Geometry check sheet. Reference: the model listing, model coordinates, mm. Face numbers are marked on the shaded views. A direction names the side the tool comes from. Round coordinates to 2 decimals unless told otherwise and drop trailing zeros. Order: outer loops, then holes, each group sorted by start corner. A loop starts at its lowest first (then second) coordinate and runs counter-clockwise, first axis right, second up. Notation, with made-up numbers: (8, 55) -> (30, 55) arc R26 cw to (30, 93) -> close; hole circle Ø5 at (61, 41). An arc over 180 degrees is marked (long way). Use a Markdown table: item, result. Add a question column.
Item 1: Material ranges on probe 1 along Y at (x, z) = (-0.25, 0); probe 2 along Y at (x, z) = (-1.5, -1.5); probe 3 along Z at (x, y) = (0, 14.25), recorded low to high. Write a range as [from, to].
Item 2: Sectioned sample at A-A, the plane y = 19.75. Record the cut outline in (x, z).
Item 3: Sectioned sample at B-B, the plane x = 0.75. Record the cut outline in (y, z).
Item 4: Set-up check for the marked faces 1 and 2: record each of +Z, -Z, +X, -X, +Y, -Y from which the full face is reachable in a straight line by a thin tool's end or side.
Item 5: Sectioned sample at C-C, the plane y = 11.5. Record the cut outline in (x, z), and give its area (3 significant figures).
Item 6: Gauge pin test, flat ends, axial feed: pin 1 Ø4 at (y, z) = (3.5, 2) entering from +X; pin 2 Ø1 at (x, y) = (0, 8) entering from +Z; pin 3 Ø1.8 at (x, z) = (-0.5, 0.5) entering from +Y. Record the tip position at first contact, or that the pin passes through.
Item 7: Sectioned sample at D-D, the plane z = 1.5. Record the cut outline in (x, y), and give its area (3 significant figures).
Item 8: Mould release check, pull along X, two halves, no side actions. Record for the marked faces 3, 4 and 5: pulls with the +X half, pulls with the -X half, needs draft (parallel to the pull), parting line crosses it, or undercut.
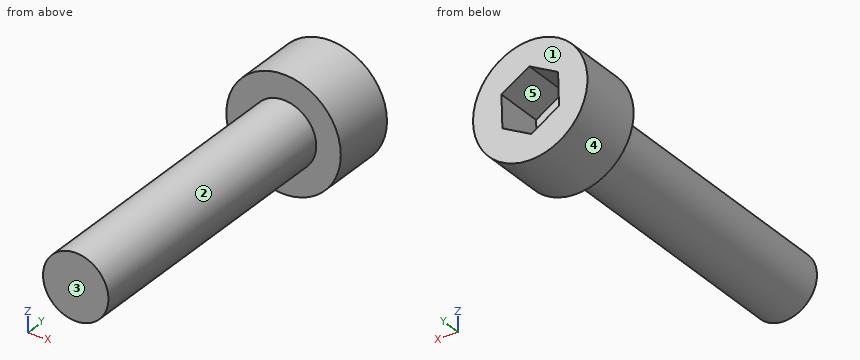
Autodesk Inventor part; units mm, degrees
ref_plane "YZ Plane" through (0, 0, 0) normal (1, 0, 0) x (0, 1, 0)
ref_plane "XZ Plane" through (0, 0, 0) normal (0, 1, 0) x (-1, 0, 0)
ref_plane "XY Plane" through (0, 0, 0) normal (0, 0, 1) x (1, 0, 0)
sketch "Sketch1" plane through (0, 0, 0) normal (0, 1, 0) x (-1, 0, 0)
  circle A0 centre (0, 0) radius 2
  dimension "d0" = 4
extrude "Extrusion1" add sketch "Sketch1" along normal blind 18
sketch "Sketch2" plane through (0, 18, 0) normal (0, 1, 0) x (1, 0, 0)
  circle A0 centre (0, 0) radius 3.5
  dimension "d5" = 7
thread "Thread1"
extrude "Extrusion2" add sketch "Sketch2" along normal blind 4
sketch "Sketch3" plane through (0, 22, 0) normal (0, 1, 0) x (1, 0, 0)
  circle A0 centre (0, 0) radius 3.5
  circle A1 centre (0, 0) radius 2
  line L0 (-1.7603, 0.9494) -> (-0.058, 1.9992)
  line L1 (-0.058, 1.9992) -> (1.7023, 1.0498)
  line L2 (1.7023, 1.0498) -> (1.7603, -0.9494)
  line L3 (1.7603, -0.9494) -> (0.058, -1.9992)
  line L4 (0.058, -1.9992) -> (-1.7023, -1.0498)
  line L5 (-1.7023, -1.0498) -> (-1.7603, 0.9494)
extrude "Extrusion3" cut sketch "Sketch3" against normal blind 3 contours L2 L3 L4 L5 L0 L1
properties part number "M4_18mm" material "Steel, Alloy"
Found:
| question | item | result |
|---|---|---|
| 1 | probe 1 | y = [0, 19] |
| 1 | probe 2 | y = [18, 22] |
| 1 | probe 3 | z = [-2, 2] |
| 2 | outline | circle Ø7 at (0, 0); hole (-1.76, -0.95) -> (-0.06, -2) -> (1.7, -1.05) -> (1.76, 0.95) -> (0.06, 2) -> (-1.7, 1.05) -> close |
| 3 | outline | (0, -1.85) -> (18, -1.85) -> (18, -3.42) -> (22, -3.42) -> (22, -1.56) -> (19, -1.56) -> (19, 1.57) -> (22, 1.57) -> (22, 3.42) -> (18, 3.42) -> (18, 1.85) -> (0, 1.85) -> close |
| 4 | face 1 | +Z, -Z, +X, -X, +Y |
| 4 | face 2 | -Y |
| 5 | outline | circle Ø4 at (0, 0) |
| 5 | area | 12.6 mm2 |
| 6 | pin 1 | stops at x = 2 |
| 6 | pin 2 | stops at z = 2 |
| 6 | pin 3 | stops at y = 19 |
| 7 | outline | (-3.16, 18) -> (-1.32, 18) -> (-1.32, 0) -> (1.32, 0) -> (1.32, 18) -> (3.16, 18) -> (3.16, 22) -> (0.87, 22) -> (0.87, 19) -> (-0.87, 19) -> (-0.87, 22) -> (-3.16, 22) -> close |
| 7 | area | 67.7 mm2 |
| 8 | face 3 | needs draft |
| 8 | face 4 | parting line crosses it |
| 8 | face 5 | undercut |
